Autodesk Inventor part; units mm, degrees
ref_plane "YZ Plane" through (0, 0, 0) normal (1, 0, 0) x (0, 1, 0)
ref_plane "XZ Plane" through (0, 0, 0) normal (0, 1, 0) x (-1, 0, 0)
ref_plane "XY Plane" through (0, 0, 0) normal (0, 0, 1) x (1, 0, 0)
sketch "Sketch1" plane through (0, 0, 0) normal (0, 0, 1) x (1, 0, 0)
  line L0 (1200, 2950) -> (-1200, 2950)
  line L1 (-1200, 2950) -> (-1200, 0)
  line L2 (-1200, 0) -> (1200, 0)
  line L3 (1200, 0) -> (1200, 2950)
  line L4 (1150, 2950) -> (1150, 0)
  line L5 (-1150, 0) -> (-1150, 2950) construction
  line L6 (0, 2950) -> (0, 50) construction
  line L7 (-1100, 200) -> (-950, 50)
  line L8 (-1200, 100) -> (-1100, 100)
  line L9 (-1100, 100) -> (-1100, 0)
  line L10 (-1100, 200) -> (-1150, 2950)
  arc A0 (-1100.4545, 224.9959) -> (-1082.3223, 182.3223) centre (-1100, 200) ccw
  arc A1 (-1082.3223, 182.3223) -> (-1100.4545, 224.9959) centre (-1100, 200) ccw construction
  line L11 (-1200, 255) -> (-1101, 255) construction
  line L12 (0, 50) -> (-950, 50)
  line L13 (0, 50) -> (0, 0)
  line L14 (1505.3449, -225.894) -> (355.3449, -225.894)
  line L15 (-1200, 245) -> (-1100.8182, 245)
  line L16 (-1200, 2900) -> (-1149.0909, 2900)
  line L17 (-1200, 999.7296) -> (-1114.5405, 999.7296)
  dimension "d3" = 2400
  dimension "d4" = 2950
  dimension "d5" = 50
  dimension "d6" = 100
  dimension "d7" = 50
  dimension "d9" = 135
  dimension "d10" = 950
  dimension "d11" = 1150
  dimension "d12" = 136.042
  dimension "d13" = 50
  dimension "d14" = 100
  dimension "d15" = 212.132
  dimension "d17" = 55
  dimension "d20" = 200
  dimension "d50" = 2705
  dimension "d53" = 50
extrude "Plate1" add sketch "Sketch1" along normal blind 3 contours L10 L17 L1 L16
sketch "Sketch2" plane through (0, 0, 3) normal (0, 0, 1) x (1, 0, 0)
  line L0 (-1149.0909, 2900) -> (-1114.5405, 999.7296)
  line L1 (-1200, 999.7296) -> (-1200, 2900)
  line L2 (-1100.8182, 245) -> (-1149.0909, 2900)
  line L3 (-1158.8362, 1267.3142) -> (-1158.778, 1264.1148)
  line L4 (-1158.778, 1264.1148) -> (-1119.3606, 1264.8314) construction
  line L5 (-1149.0909, 2900) -> (-1100.8182, 245)
  line L6 (-1158.778, 1264.1148) -> (-1200, 1263.3653)
  line L7 (-1158.8362, 1267.3142) -> (-1200, 1266.5658)
  line L8 (-1200, 703.2727) -> (-1153.6813, 704.1149)
  line L9 (-1153.6813, 704.1149) -> (-1153.7395, 707.3144)
  line L10 (-1153.6813, 704.1149) -> (-1109.1804, 704.924) construction
  line L11 (-1153.7395, 707.3144) -> (-1200, 706.4732)
  line L12 (-1200, 1823.4578) -> (-1163.8614, 1824.1149)
  line L13 (-1163.8614, 1824.1149) -> (-1163.9196, 1827.3144)
  line L14 (-1163.9196, 1827.3144) -> (-1200, 1826.6584)
  line L15 (-1163.8614, 1824.1149) -> (-1129.5407, 1824.7389) construction
  line L16 (-1200, 2383.5504) -> (-1168.9515, 2384.1149)
  line L17 (-1168.9515, 2384.1149) -> (-1169.0097, 2387.3144)
  line L18 (-1168.9515, 2384.1149) -> (-1139.7208, 2384.6464) construction
  line L19 (-1169.0097, 2387.3144) -> (-1200, 2386.7509)
  line L20 (-1200, 2900) -> (-1149.0909, 2900)
  line L21 (-1114.5405, 999.7296) -> (-1200, 999.7296)
  point P0 (0, 0)
  point P1 (-1150, 2950)
  dimension "d34" = 46.3264
  dimension "d36" = 41.2288
  dimension "d39" = 36.1445
  dimension "d42" = 31.0536
  dimension "d43" = 560
  dimension "d44" = 3.2
  dimension "d45" = 560
  dimension "d46" = 3.2
  dimension "d47" = 560
  dimension "d48" = 3.2
  dimension "d49" = 3.2
  dimension "d52" = 460
extrude "Extrusion1" cut sketch "Sketch2" against normal through all contours L19 L17 L16 L1 | L1 L7 L3 L6 | L14 L13 L12 L1
sketch "Sketch3" plane through (0, 0, 0) normal (0, 0, -1) x (-1, 0, 0)
  line L0 (1163.9196, 1827.3144) -> (1200, 1826.6584) construction
  line L1 (1200, 2383.5504) -> (1200, 1826.6584) construction
  line L2 (1200, 2383.5504) -> (1168.9515, 2384.1149) construction
  line L3 (1168.9515, 2384.1149) -> (1169.0097, 2387.3144) construction
  line L4 (1169.0097, 2387.3144) -> (1200, 2386.7509) construction
  line L5 (1200, 2900) -> (1200, 2386.7509) construction
  line L6 (1149.0909, 2900) -> (1200, 2900) construction
  line L7 (1200, 1263.3653) -> (1158.778, 1264.1148) construction
  line L8 (1158.778, 1264.1148) -> (1158.8362, 1267.3142) construction
  line L9 (1158.8362, 1267.3142) -> (1200, 1266.5658) construction
  line L10 (1200, 1823.4578) -> (1200, 1266.5658) construction
  line L11 (1200, 1823.4578) -> (1163.8614, 1824.1149) construction
  line L12 (1163.8614, 1824.1149) -> (1163.9196, 1827.3144) construction
  line L13 (1130.7428, 1027.3062) -> (1187.6517, 1027.3062) construction
  line L14 (1187.6517, 1027.3062) -> (1187.6517, 1023.7324) construction
  line L15 (1187.6517, 1023.7324) -> (1130.7428, 1023.7324) construction
  line L16 (1130.7428, 1023.7324) -> (1130.7428, 1027.3062) construction
  point P0 (0, 0)
mark "Mark1"
equation "\"d11\" = d10 + d18"
equation "\"d14\" = d6"
equation "\"d43\" = Stringer1_step"
equation "\"d45\" = Stringer1_step"
equation "\"d47\" = Stringer1_step"
equation "\"d52\" = Stringer1_hight"
equation "\"d2\" = Thickness"
equation "\"BendReliefWidth\" = Thickness"
equation "\"BendReliefDepth\" = 0.5 * Thickness"
equation "\"CornerReliefSize\" = 4 * Thickness"
equation "\"MinimumRemnant\" = 2 * Thickness"
equation "\"TransitionRadius\" = BendRadius"
equation "\"JacobiRadiusSize\" = BendRadius"
equation "\"GapSize\" = Thickness"
equation "\"d18\" = d19"
properties part number "BSH 024 rib board short" material "09g2s"
Model file for the job. Use its own axes, mm. Coordinates: 2 decimals unless noted, no trailing zeros. Loops run counter-clockwise (first coordinate to the right, second up) from the corner with the lowest first, then second, coordinate; pieces in that order, holes last. Notation, with made-up numbers: (-5.5, -28) - (52.5, -28) arc R4 ccw to (52.5, -23) - close; hole circle Ø11 at (-30, 25). An arc over 180 degrees is marked (long way). Answer as a JSON object with one key per item and string values. Group by question number.
(1) Cut at B-B (y = 2247). Give the cut face in (x, z).
(2) Cut at A-A (z = 1.1). Give the cut face in (x, y).
(3) Probe line 1 along Y through (x, z) = (-1180.5, 0.5); line 2 along Y through (x, z) = (-1176, 1.95); line 3 along Y through (x, z) = (-1160, 2.75). List the from-to ranges inside material, lowest first.
(4) Flat gauge pins, fed straight in: pin 1 (2 mm diameter, centred on x = -1187, y = 2252, fed in from -Z); pin 2 (1 mm diameter, centred on y = 1667, z = 2.5, fed in from +X); pin 3 (1 mm diameter, centred on y = 2680.5, z = 1.5, fed in from +X). Where does each tip first touch, or does it go through?
(5) Cut at C-C (y = 2645). Give the cut face in (x, z).
Geometry says:
{
 "1": {"outline": "(-1200, 0) - (-1137.22, 0) - (-1137.22, 3) - (-1200, 3) - close"},
 "2": {"outline": "(-1200, 999.73) - (-1114.54, 999.73) - (-1149.09, 2900) - (-1200, 2900) - (-1200, 2386.75) - (-1169.01, 2387.31) - (-1168.95, 2384.11) - (-1200, 2383.55) - (-1200, 1826.66) - (-1163.92, 1827.31) - (-1163.86, 1824.11) - (-1200, 1823.46) - (-1200, 1266.57) - (-1158.84, 1267.31) - (-1158.78, 1264.11) - (-1200, 1263.37) - close"},
 "3": {"line 1": "y = 999.73 to 1263.72, 1266.92 to 1823.81, 1827.01 to 2383.9, 2387.11 to 2900", "line 2": "y = 999.73 to 1263.8, 1267 to 1823.89, 1827.09 to 2383.99, 2387.19 to 2900", "line 3": "y = 999.73 to 1264.09, 1267.29 to 2900"},
 "4": {"pin 1": "stops at z = 0", "pin 2": "stops at x = -1126.66", "pin 3": "stops at x = -1145.09"},
 "5": {"outline": "(-1200, 0) - (-1144.45, 0) - (-1144.45, 3) - (-1200, 3) - close"}
}
